The listing builds one solid part. Answer for the finished solid, in the listing's coordinates (mm). Coordinates: 2 decimals unless noted, no trailing zeros. Write each loop counter-clockwise with the first axis right and the second up, starting at its lowest first coordinate (ties: lowest second). Pieces come first, ordered by that corner, then holes.
(1) Straight lines are drawn through the part: line 1 (X direction, y = 1.35, z = 0) (3 decimals); line 2 (Z direction, x = -6.5, y = 1.9); line 3 (Z direction, x = -11, y = 2.9). For each, find the intervals that lie inside material, in ascending order.
(2) The part is cut by section B-B on x = 51.25. Determine the outline of the cut face in (y, z) (3 decimals), plus the area to 3 significant figures.
(3) The part is cut by section C-C on z = 40.5. Determine the outline of the cut face in (x, y) (3 decimals).
(4) The part is cut by section A-A on z = 57.15. Determine the outline of the cut face in (x, y) (3 decimals), plus the area to 3 significant figures.
(5) The part is cut by section D-D on x = -57.15. Determine the outline of the cut face in (y, z) (3 decimals).
(6) Given P1, Ø1, axis at x = -10.5, y = 1.5, coming from the -Z side; P2, Ø4.5, axis at x = 0, z = -57.15, coming from the +Y side (3 decimals), each flat-ended and moving along its own axis, determine where each tip first touches the part or whether it passes through.
from build123d import *

# Parameters (mm, degrees)
SKETCH1_R                 = 69.85
PLATE_DEPTH               = 3.175
PLATE_CENTER_HOLE_REACH   = 100.834
SKETCH2_R                 = 12.7
PLATE_THROUGH_HOLES_REACH = 100.834
SKETCH13_R                = 1.875
SKETCH13_R_2              = 1.5
SKETCH13_R_3              = 9.5


with BuildPart() as part:
    # Sketch1 → plate (new body)
    with BuildSketch(Plane(origin=(0, 0, 0), x_dir=(1, 0, 0), z_dir=(0, 1, 0))):
        with Locations(Location((0, 0, 0), (0, 0, 270))):
            Circle(SKETCH1_R)
    extrude(amount=PLATE_DEPTH)

    # Sketch2 → plate center hole (cut, up to next)
    with BuildSketch(Plane.XZ, mode=Mode.PRIVATE) as plate_center_hole_sk1:
        with Locations(Location((0, 0, 0), (0, 0, 270))):
            Circle(SKETCH2_R)
    plate_center_hole_tool1 = extrude(plate_center_hole_sk1.sketch, amount=-PLATE_CENTER_HOLE_REACH, mode=Mode.PRIVATE) & part.part
    add(plate_center_hole_tool1.solids().sort_by_distance((0, 0, 0))[0], mode=Mode.SUBTRACT)

    # Sketch13 → plate through holes (cut, up to next)
    with BuildSketch(Plane.XZ, mode=Mode.PRIVATE) as plate_through_holes_sk1:
        with Locations(Location((-12.25, 25, 0), (0, 0, 270))):
            Circle(SKETCH13_R)
    plate_through_holes_tool1 = extrude(plate_through_holes_sk1.sketch, amount=-PLATE_THROUGH_HOLES_REACH, mode=Mode.PRIVATE) & part.part
    # Sketch13 → plate through holes (cut, up to next)
    with BuildSketch(Plane.XZ, mode=Mode.PRIVATE) as plate_through_holes_sk2:
        with Locations(Location((-51.25, 25, 0), (0, 0, 90))):
            Circle(SKETCH13_R)
    plate_through_holes_tool2 = extrude(plate_through_holes_sk2.sketch, amount=-PLATE_THROUGH_HOLES_REACH, mode=Mode.PRIVATE) & part.part
    # Sketch13 → plate through holes (cut, up to next)
    with BuildSketch(Plane.XZ, mode=Mode.PRIVATE) as plate_through_holes_sk3:
        with Locations(Location((-51.25, -25, 0), (0, 0, 270))):
            Circle(SKETCH13_R)
    plate_through_holes_tool3 = extrude(plate_through_holes_sk3.sketch, amount=-PLATE_THROUGH_HOLES_REACH, mode=Mode.PRIVATE) & part.part
    # Sketch13 → plate through holes (cut, up to next)
    with BuildSketch(Plane.XZ, mode=Mode.PRIVATE) as plate_through_holes_sk4:
        with Locations(Location((-12.25, -25, 0), (0, 0, 90))):
            Circle(SKETCH13_R)
    plate_through_holes_tool4 = extrude(plate_through_holes_sk4.sketch, amount=-PLATE_THROUGH_HOLES_REACH, mode=Mode.PRIVATE) & part.part
    # Sketch13 → plate through holes (cut, up to next)
    with BuildSketch(Plane.XZ, mode=Mode.PRIVATE) as plate_through_holes_sk5:
        with Locations(Location((12.25, -25, 0), (0, 0, 270))):
            Circle(SKETCH13_R)
    plate_through_holes_tool5 = extrude(plate_through_holes_sk5.sketch, amount=-PLATE_THROUGH_HOLES_REACH, mode=Mode.PRIVATE) & part.part
    # Sketch13 → plate through holes (cut, up to next)
    with BuildSketch(Plane.XZ, mode=Mode.PRIVATE) as plate_through_holes_sk6:
        with Locations(Location((51.25, -25, 0), (0, 0, 90))):
            Circle(SKETCH13_R)
    plate_through_holes_tool6 = extrude(plate_through_holes_sk6.sketch, amount=-PLATE_THROUGH_HOLES_REACH, mode=Mode.PRIVATE) & part.part
    # Sketch13 → plate through holes (cut, up to next)
    with BuildSketch(Plane.XZ, mode=Mode.PRIVATE) as plate_through_holes_sk7:
        with Locations(Location((51.25, 25, 0), (0, 0, 270))):
            Circle(SKETCH13_R)
    plate_through_holes_tool7 = extrude(plate_through_holes_sk7.sketch, amount=-PLATE_THROUGH_HOLES_REACH, mode=Mode.PRIVATE) & part.part
    # Sketch13 → plate through holes (cut, up to next)
    with BuildSketch(Plane.XZ, mode=Mode.PRIVATE) as plate_through_holes_sk8:
        with Locations(Location((12.25, 25, 0), (0, 0, 90))):
            Circle(SKETCH13_R)
    plate_through_holes_tool8 = extrude(plate_through_holes_sk8.sketch, amount=-PLATE_THROUGH_HOLES_REACH, mode=Mode.PRIVATE) & part.part
    # Sketch13 → plate through holes (cut, up to next)
    with BuildSketch(Plane.XZ, mode=Mode.PRIVATE) as plate_through_holes_sk9:
        with Locations(Location((57.15, 0, 0), (0, 0, 270))):
            Circle(SKETCH13_R)
    plate_through_holes_tool9 = extrude(plate_through_holes_sk9.sketch, amount=-PLATE_THROUGH_HOLES_REACH, mode=Mode.PRIVATE) & part.part
    # Sketch13 → plate through holes (cut, up to next)
    with BuildSketch(Plane.XZ, mode=Mode.PRIVATE) as plate_through_holes_sk10:
        with Locations(Location((40.411152545, 40.411152545, 0), (0, 0, 270))):
            Circle(SKETCH13_R)
    plate_through_holes_tool10 = extrude(plate_through_holes_sk10.sketch, amount=-PLATE_THROUGH_HOLES_REACH, mode=Mode.PRIVATE) & part.part
    # Sketch13 → plate through holes (cut, up to next)
    with BuildSketch(Plane.XZ, mode=Mode.PRIVATE) as plate_through_holes_sk11:
        with Locations(Location((40.411152545, -40.411152545, 0), (0, 0, 270))):
            Circle(SKETCH13_R)
    plate_through_holes_tool11 = extrude(plate_through_holes_sk11.sketch, amount=-PLATE_THROUGH_HOLES_REACH, mode=Mode.PRIVATE) & part.part
    # Sketch13 → plate through holes (cut, up to next)
    with BuildSketch(Plane.XZ, mode=Mode.PRIVATE) as plate_through_holes_sk12:
        with Locations(Location((0, -57.15, 0), (0, 0, 270))):
            Circle(SKETCH13_R)
    plate_through_holes_tool12 = extrude(plate_through_holes_sk12.sketch, amount=-PLATE_THROUGH_HOLES_REACH, mode=Mode.PRIVATE) & part.part
    # Sketch13 → plate through holes (cut, up to next)
    with BuildSketch(Plane.XZ, mode=Mode.PRIVATE) as plate_through_holes_sk13:
        with Locations(Location((-40.411152545, -40.411152545, 0), (0, 0, 270))):
            Circle(SKETCH13_R)
    plate_through_holes_tool13 = extrude(plate_through_holes_sk13.sketch, amount=-PLATE_THROUGH_HOLES_REACH, mode=Mode.PRIVATE) & part.part
    # Sketch13 → plate through holes (cut, up to next)
    with BuildSketch(Plane.XZ, mode=Mode.PRIVATE) as plate_through_holes_sk14:
        with Locations(Location((-57.15, 0, 0), (0, 0, 270))):
            Circle(SKETCH13_R)
    plate_through_holes_tool14 = extrude(plate_through_holes_sk14.sketch, amount=-PLATE_THROUGH_HOLES_REACH, mode=Mode.PRIVATE) & part.part
    # Sketch13 → plate through holes (cut, up to next)
    with BuildSketch(Plane.XZ, mode=Mode.PRIVATE) as plate_through_holes_sk15:
        with Locations(Location((-40.411152545, 40.411152545, 0), (0, 0, 270))):
            Circle(SKETCH13_R)
    plate_through_holes_tool15 = extrude(plate_through_holes_sk15.sketch, amount=-PLATE_THROUGH_HOLES_REACH, mode=Mode.PRIVATE) & part.part
    # Sketch13 → plate through holes (cut, up to next)
    with BuildSketch(Plane.XZ, mode=Mode.PRIVATE) as plate_through_holes_sk16:
        with Locations(Location((0, 57.15, 0), (0, 0, 270))):
            Circle(SKETCH13_R)
    plate_through_holes_tool16 = extrude(plate_through_holes_sk16.sketch, amount=-PLATE_THROUGH_HOLES_REACH, mode=Mode.PRIVATE) & part.part
    # Sketch13 → plate through holes (cut, up to next)
    with BuildSketch(Plane.XZ, mode=Mode.PRIVATE) as plate_through_holes_sk17:
        with Locations(Location((-29, -24.5, 0), (0, 0, 270))):
            Circle(SKETCH13_R_2)
    plate_through_holes_tool17 = extrude(plate_through_holes_sk17.sketch, amount=-PLATE_THROUGH_HOLES_REACH, mode=Mode.PRIVATE) & part.part
    # Sketch13 → plate through holes (cut, up to next)
    with BuildSketch(Plane.XZ, mode=Mode.PRIVATE) as plate_through_holes_sk18:
        with Locations(Location((-29, 24.5, 0), (0, 0, 90))):
            Circle(SKETCH13_R_2)
    plate_through_holes_tool18 = extrude(plate_through_holes_sk18.sketch, amount=-PLATE_THROUGH_HOLES_REACH, mode=Mode.PRIVATE) & part.part
    # Sketch13 → plate through holes (cut, up to next)
    with BuildSketch(Plane.XZ, mode=Mode.PRIVATE) as plate_through_holes_sk19:
        with Locations(Location((29, 24.5, 0), (0, 0, 270))):
            Circle(SKETCH13_R_2)
    plate_through_holes_tool19 = extrude(plate_through_holes_sk19.sketch, amount=-PLATE_THROUGH_HOLES_REACH, mode=Mode.PRIVATE) & part.part
    # Sketch13 → plate through holes (cut, up to next)
    with BuildSketch(Plane.XZ, mode=Mode.PRIVATE) as plate_through_holes_sk20:
        with Locations(Location((29, -24.5, 0), (0, 0, 90))):
            Circle(SKETCH13_R_2)
    plate_through_holes_tool20 = extrude(plate_through_holes_sk20.sketch, amount=-PLATE_THROUGH_HOLES_REACH, mode=Mode.PRIVATE) & part.part
    # Sketch13 → plate through holes (cut, up to next)
    with BuildSketch(Plane.XZ, mode=Mode.PRIVATE) as plate_through_holes_sk21:
        with Locations(Location((0, -40, 0), (0, 0, 270))):
            Circle(SKETCH13_R_3)
    plate_through_holes_tool21 = extrude(plate_through_holes_sk21.sketch, amount=-PLATE_THROUGH_HOLES_REACH, mode=Mode.PRIVATE) & part.part
    add(plate_through_holes_tool1.solids().sort_by_distance((-12.25, 0, 25))[0], mode=Mode.SUBTRACT)
    add(plate_through_holes_tool2.solids().sort_by_distance((-51.25, 0, 25))[0], mode=Mode.SUBTRACT)
    add(plate_through_holes_tool3.solids().sort_by_distance((-51.25, 0, -25))[0], mode=Mode.SUBTRACT)
    add(plate_through_holes_tool4.solids().sort_by_distance((-12.25, 0, -25))[0], mode=Mode.SUBTRACT)
    add(plate_through_holes_tool5.solids().sort_by_distance((12.25, 0, -25))[0], mode=Mode.SUBTRACT)
    add(plate_through_holes_tool6.solids().sort_by_distance((51.25, 0, -25))[0], mode=Mode.SUBTRACT)
    add(plate_through_holes_tool7.solids().sort_by_distance((51.25, 0, 25))[0], mode=Mode.SUBTRACT)
    add(plate_through_holes_tool8.solids().sort_by_distance((12.25, 0, 25))[0], mode=Mode.SUBTRACT)
    add(plate_through_holes_tool9.solids().sort_by_distance((57.15, 0, 0))[0], mode=Mode.SUBTRACT)
    add(plate_through_holes_tool10.solids().sort_by_distance((40.411153, 0, 40.411153))[0], mode=Mode.SUBTRACT)
    add(plate_through_holes_tool11.solids().sort_by_distance((40.411153, 0, -40.411153))[0], mode=Mode.SUBTRACT)
    add(plate_through_holes_tool12.solids().sort_by_distance((0, 0, -57.15))[0], mode=Mode.SUBTRACT)
    add(plate_through_holes_tool13.solids().sort_by_distance((-40.411153, 0, -40.411153))[0], mode=Mode.SUBTRACT)
    add(plate_through_holes_tool14.solids().sort_by_distance((-57.15, 0, 0))[0], mode=Mode.SUBTRACT)
    add(plate_through_holes_tool15.solids().sort_by_distance((-40.411153, 0, 40.411153))[0], mode=Mode.SUBTRACT)
    add(plate_through_holes_tool16.solids().sort_by_distance((0, 0, 57.15))[0], mode=Mode.SUBTRACT)
    add(plate_through_holes_tool17.solids().sort_by_distance((-29, 0, -24.5))[0], mode=Mode.SUBTRACT)
    add(plate_through_holes_tool18.solids().sort_by_distance((-29, 0, 24.5))[0], mode=Mode.SUBTRACT)
    add(plate_through_holes_tool19.solids().sort_by_distance((29, 0, 24.5))[0], mode=Mode.SUBTRACT)
    add(plate_through_holes_tool20.solids().sort_by_distance((29, 0, -24.5))[0], mode=Mode.SUBTRACT)
    add(plate_through_holes_tool21.solids().sort_by_distance((0, 0, -40))[0], mode=Mode.SUBTRACT)


solid = part.part
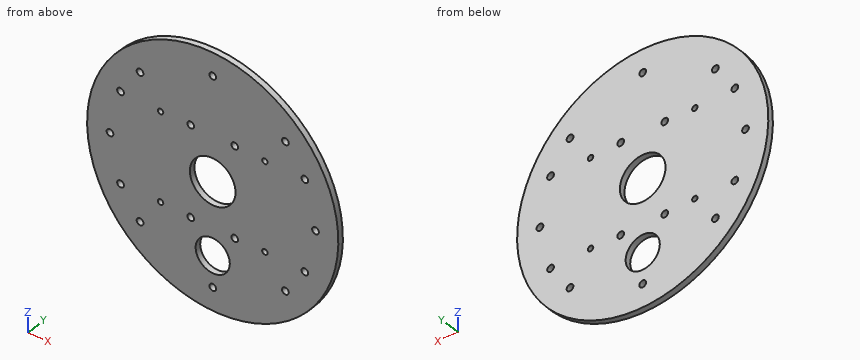
Model answer:
1. line 1: x = -69.85 to -59.025, -55.275 to -12.7, 12.7 to 55.275, 59.025 to 69.85
1. line 2: z = -69.55 to -46.93, -33.07 to -10.91, 10.91 to 69.55
1. line 3: z = -68.98 to -26.4, -23.6 to -6.35, 6.35 to 23.6, 26.4 to 68.98
2. outline: (0, -47.46) - (3.175, -47.46) - (3.175, -26.875) - (0, -26.875) - close; (0, -23.125) - (3.175, -23.125) - (3.175, 23.125) - (0, 23.125) - close; (0, 26.875) - (3.175, 26.875) - (3.175, 47.46) - (0, 47.46) - close
2. area: 278 mm2
3. outline: (-56.91, 0) - (-42.284, 0) - (-42.284, 3.175) - (-56.91, 3.175) - close; (-38.538, 0) - (38.538, 0) - (38.538, 3.175) - (-38.538, 3.175) - close; (42.284, 0) - (56.91, 0) - (56.91, 3.175) - (42.284, 3.175) - close
4. outline: (-40.161, 0) - (-1.875, 0) - (-1.875, 3.175) - (-40.161, 3.175) - close; (1.875, 0) - (40.161, 0) - (40.161, 3.175) - (1.875, 3.175) - close
4. area: 243 mm2
5. outline: (0, -40.161) - (3.175, -40.161) - (3.175, -1.875) - (0, -1.875) - close; (0, 1.875) - (3.175, 1.875) - (3.175, 40.161) - (0, 40.161) - close
6. P1: stops at z = -69.13
6. P2: stops at y = 3.175
